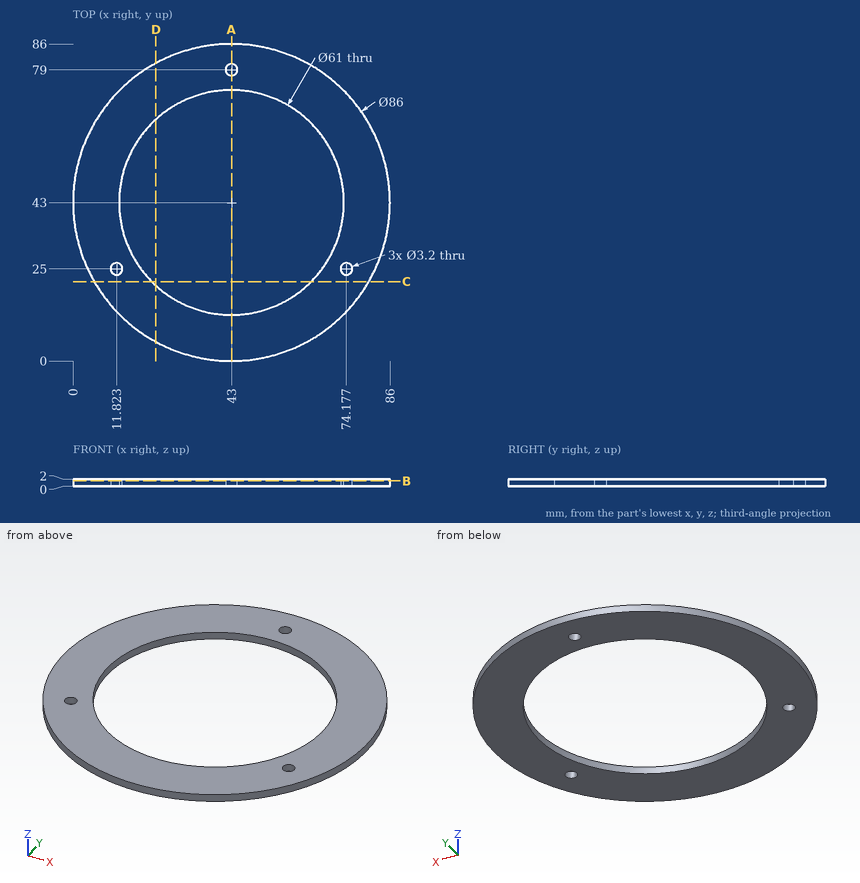
Can you work these out from the drawing? Everything is in mm from the part's minimum corner. Round coordinates to 2 decimals unless told otherwise and drop trailing zeros. Loops run counter-clockwise (first coordinate to the right, second up) from the corner with the lowest first, then second, coordinate; pieces in that order, holes last. Notation, with made-up numbers: (33.5, -9.75) - (41.5, -9.75) arc R16 ccw to (41.5, -4.75) - close; hole circle Ø5 at (66.5, 63). An arc over 180 degrees is marked (long way). One line per question, with ' | ' between items. Start each with the question number.
Q1. I want a section at D-D (x = 22.5). Write out the boundary of the cut face in (y, z).
Q2. I want a section at B-B (z = 1.5). Write out the boundary of the cut face in (x, y).
Q3. Please list where these lines run through material, in increasing order: line 1 (Y direction, x = 43, z = 1.6); line 2 (X direction, y = 44, z = 1.4); line 3 (Y direction, x = 31, z = 0.95). Write a range as [from, to].
Q4. I want a section at C-C (y = 21.5). Write out the boundary of the cut face in (x, z), then the cut area to 3 significant figures.
Q5. I want a section at A-A (x = 43). Write out the boundary of the cut face in (y, z), then the cut area to 3 significant figures.
Q6. Will this pin go through, and if not, where does the flat tip stop? pin 1 (2.5 mm diameter, centred on x = 11.82, y = 25, fed in from -Z).
Response values:
1) outline: (5.2, 0) - (20.42, 0) - (20.42, 2) - (5.2, 2) - close; (65.58, 0) - (80.8, 0) - (80.8, 2) - (65.58, 2) - close
2) outline: circle Ø86 at (43, 43); hole circle Ø3.2 at (11.82, 25); hole circle Ø61 at (43, 43); hole circle Ø3.2 at (43, 79); hole circle Ø3.2 at (74.18, 25)
3) line 1: y = [0, 12.5], [73.5, 77.4], [80.6, 86] | line 2: x = [0.01, 12.52], [73.48, 85.99] | line 3: y = [1.71, 14.96], [71.04, 84.29]
4) outline: (5.76, 0) - (21.37, 0) - (21.37, 2) - (5.76, 2) - close; (64.63, 0) - (80.24, 0) - (80.24, 2) - (64.63, 2) - close | area: 62.4 mm²
5) outline: (0, 0) - (12.5, 0) - (12.5, 2) - (0, 2) - close; (73.5, 0) - (77.4, 0) - (77.4, 2) - (73.5, 2) - close; (80.6, 0) - (86, 0) - (86, 2) - (80.6, 2) - close | area: 43.6 mm²
6) pin 1: passes through
